from build123d import *

# Parameters (mm, degrees)
SKETCH1_R               = 45
SKETCH1_R_2             = 44
BOSS_EXTRUDE1_DEPTH     = 18
BOSS_EXTRUDE2_START     = -2
SKETCH1_2_R             = 45
SKETCH1_2_R_2           = 44
BOSS_EXTRUDE2_DEPTH     = 2
M3_5X0_6_TAPPED_HOLE1_D = 2.9
CIRPATTERN1_COUNT       = 4
CUT_EXTRUDE1_DEPTH      = 67.708320321
CUT_EXTRUDE1_DEPTH_BACK = 67.708320321
SKETCH2_R               = 10


with BuildPart() as part:
    # Sketch1 → Boss-Extrude1 (new body)
    with BuildSketch(Plane.XY):
        Circle(SKETCH1_R)
        Circle(SKETCH1_R_2, mode=Mode.SUBTRACT)
    extrude(amount=BOSS_EXTRUDE1_DEPTH)

    # Sketch1<2> → Boss-Extrude2 (add)
    # profile 1 of 2: a face of its own
    with BuildSketch(Plane.XY.offset(BOSS_EXTRUDE2_START)):
        Circle(SKETCH1_2_R)
        Circle(SKETCH1_2_R_2, mode=Mode.SUBTRACT)
    # profile 2 of 2: a face of its own
    with BuildSketch(Plane.XY.offset(BOSS_EXTRUDE2_START)):
        Circle(SKETCH1_2_R_2)
    extrude(amount=BOSS_EXTRUDE2_DEPTH)

    # M3.5x0.6 Tapped Hole1 (through all)
    with Locations(Plane(origin=(0, 0, -2), x_dir=(-1, 0, 0), z_dir=(0, 0, -1))):
        with Locations((10.960155108, 10.960155108)):
            m3_5x0_6_tapped_hole1 = Hole(M3_5X0_6_TAPPED_HOLE1_D / 2)

    # CirPattern1: M3.5x0.6 Tapped Hole1 ×4 about axis
    cirpattern1_axis = Axis((0.011391445, -0.011391445, 0), (0, 0, 1))
    for i in range(1, CIRPATTERN1_COUNT):
        add(m3_5x0_6_tapped_hole1.rotate(cirpattern1_axis, i * 360 / CIRPATTERN1_COUNT), mode=Mode.SUBTRACT)

    # Sketch2 → Cut-Extrude1 (cut, two sides: drawn at the far end of the back side and taken through both)
    with BuildSketch(Plane(origin=(0, 0, -2), x_dir=(-1, 0, 0), z_dir=(0, 0, -1)).offset(-CUT_EXTRUDE1_DEPTH_BACK)):
        with Locations(Location((0, 0, 0), (0, 0, 180))):
            Circle(SKETCH2_R)
    extrude(amount=CUT_EXTRUDE1_DEPTH + CUT_EXTRUDE1_DEPTH_BACK, mode=Mode.SUBTRACT)


solid = part.part
Geometry: final body of the model. Coordinates: model frame, mm. A direction names the side the tool comes from. Give positions to 0.01 mm unless a question says otherwise; leave off trailing zeros. Order: outer loops, then holes, each group sorted by start corner. A loop starts at its lowest first (then second) coordinate and runs counter-clockwise, first axis right, second up. Notation, with made-up numbers: (-34, 12.25) -> (9, 12.25) arc R12 cw to (9, 32.25) -> close; hole circle Ø11 at (-15.5, -32). An arc over 180 degrees is marked (long way). Write each question's results on one line, items separated by ' | '.
1) Draft query along X for faces 1 (the face through (-10, 0, -1)), 2 (the face through (20.765, -39.923, 7.86)), 3 (the face through (43.1, -9.8, 18)), 4 (the face through (-12.11, 10.08, -0.99)). Return one class per face: released by +X, released by -X, zero draft, split by the parting line, or undercut.
Geometry says:
face 1: undercut | face 2: split by the parting line | face 3: zero draft | face 4: undercut
2) Cut plane C-C (x = -22). Output: boundary loops of the cut face in (y, z).
Geometry says:
outline: (-39.26, -2) -> (39.26, -2) -> (39.26, 18) -> (38.11, 18) -> (38.11, 0) -> (-38.11, 0) -> (-38.11, 18) -> (-39.26, 18) -> close
3) Cut plane D-D (y = -19.5). Output: boundary loops of the cut face in (x, z), and give its area (3 significant figures).
Geometry says:
outline: (-40.56, -2) -> (40.56, -2) -> (40.56, 18) -> (39.44, 18) -> (39.44, 0) -> (-39.44, 0) -> (-39.44, 18) -> (-40.56, 18) -> close | area: 202 mm²
4) Line query: line 1 along Y through (x, z) = (0, 12.5); line 2 along Z through (x, y) = (-10, -14); line 3 along Y through (x, z) = (3.5, 6.25). Output: solid intervals per line, ascending.
Geometry says:
line 1: y = -45 to -44, 44 to 45 | line 2: z = -2 to 0 | line 3: y = -44.86 to -43.86, 43.86 to 44.86
5) Cut plane A-A (x = 0). Output: boundary loops of the cut face in (y, z).
Geometry says:
outline: (-45, -2) -> (-10, -2) -> (-10, 0) -> (-44, 0) -> (-44, 18) -> (-45, 18) -> close; (10, -2) -> (45, -2) -> (45, 18) -> (44, 18) -> (44, 0) -> (10, 0) -> close
6) First-contact query: pin 1 Ø2 at (y, z) = (4, 11) entering from +X; pin 2 Ø23 at (x, y) = (0, 0) entering from +Z; pin 3 Ø8 at (x, z) = (-23, 10.5) entering from -Y. Flat tips, straight axial feed; report the tip coordinate or a pass-through.
Geometry says:
pin 1: stops at x = 44.9 | pin 2: stops at z = 0 | pin 3: stops at y = -40.79
7) Set-up query: faces 5 (the face through (-10.4, 0.6, 0)), 6 (the face through (-1, 11, -2)). Return all of +Z, -Z, +X, -X, +Y, -Y with unobstructed straight access to the full face (end or side cutting, diameter ignored); none if empty.
Geometry says:
face 5: +Z | face 6: -Z, +X, -X, +Y, -Y
